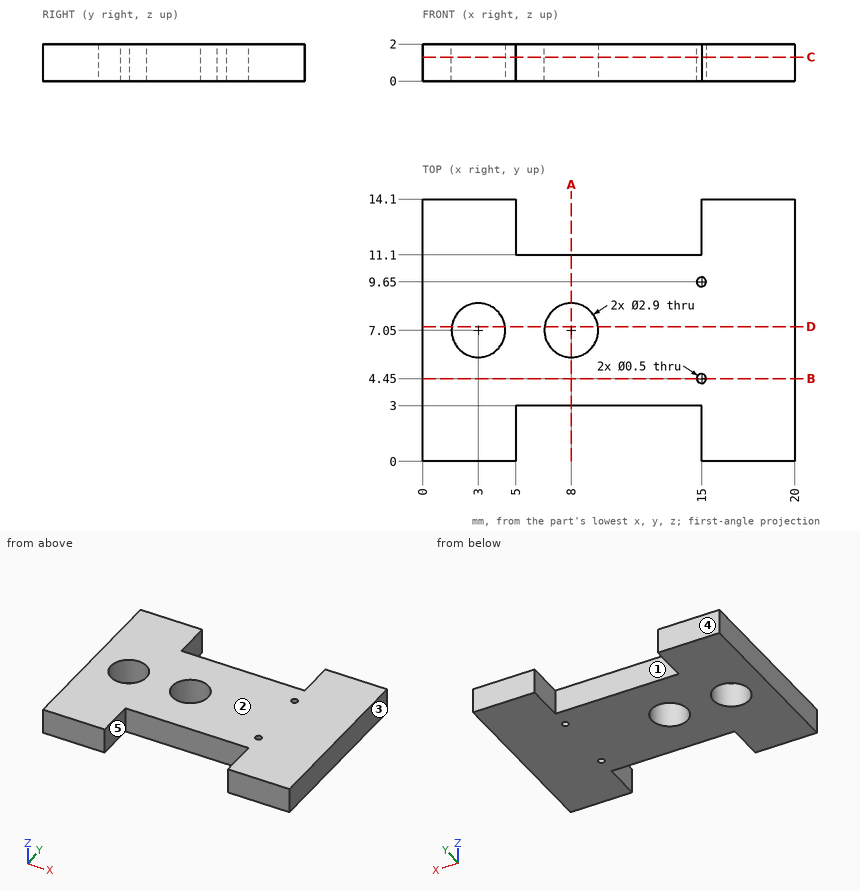
Geometry check sheet. Reference: drawing and pictorial views, mm from the part's lowest x, y, z. A direction names the side the tool comes from. Give positions to 0.01 mm unless a question says otherwise; leave off trailing zeros. Order: outer loops, then holes, each group sorted by start corner. A loop starts at its lowest first (then second) coordinate and runs counter-clockwise, first axis right, second up.
1. Access from +Z, -Z, +X, -X, +Y, -Y to the whole of each face (thin tool, end or side, straight path). Record for the marked faces 4 and 5.
2. Section check A-A, the plane x = 8. Enter the section's corners in (y, z).
3. Section check C-C, the plane z = 1.3. Enter the section's corners in (x, y), and give its area (3 significant figures).
4. Section check D-D, the plane y = 7.25. Enter the section's corners in (x, z).
5. Release check for a two-part mould opening along X. For the marked faces 1, 2 and 3 record: pulls with the +X half, pulls with the -X half, needs draft (parallel to the pull), parting line crosses it, or undercut.
6. Thickness scan on L1, parallel to Y at x = 3, z = 0.6; L2, parallel to Y at x = 8, z = 1.25; L3, parallel to X at y = 2.5, z = 0.3. Record the ranges inside material, lowest first.
7. Section check B-B, the plane y = 4.45. Enter the section's corners in (x, z), and give its area (3 significant figures).
8. Gauge pin test, flat end, axial feed: pin 1 Ø1 at (x, z) = (8.5, 1) entering from +Y. Record the tip position at first contact, or that the pin passes through.
Values follow:
1. face 4: +Z, -Z, +X, -X, +Y
1. face 5: +Z, -Z, -Y
2. outline: (3, 0) - (5.6, 0) - (5.6, 2) - (3, 2) - close; (8.5, 0) - (11.1, 0) - (11.1, 2) - (8.5, 2) - close
3. outline: (0, 0) - (5, 0) - (5, 3) - (15, 3) - (15, 0) - (20, 0) - (20, 14.1) - (15, 14.1) - (15, 11.1) - (5, 11.1) - (5, 14.1) - (0, 14.1) - close; hole circle Ø2.9 at (3, 7.05); hole circle Ø2.9 at (8, 7.05); hole circle Ø0.5 at (15, 4.45); hole circle Ø0.5 at (15, 9.65)
3. area: 208 mm2
4. outline: (0, 0) - (1.56, 0) - (1.56, 2) - (0, 2) - close; (4.44, 0) - (6.56, 0) - (6.56, 2) - (4.44, 2) - close; (9.44, 0) - (20, 0) - (20, 2) - (9.44, 2) - close
5. face 1: undercut
5. face 2: needs draft
5. face 3: pulls with the +X half
6. L1: y = 0 to 5.6, 8.5 to 14.1
6. L2: y = 3 to 5.6, 8.5 to 11.1
6. L3: x = 0 to 5, 15 to 20
7. outline: (0, 0) - (14.75, 0) - (14.75, 2) - (0, 2) - close; (15.25, 0) - (20, 0) - (20, 2) - (15.25, 2) - close
7. area: 39.0 mm2
8. pin 1: stops at y = 11.1
